```python
from build123d import *

# Parameters (mm, degrees)
ESQUISSE1_W        = 117.07
ESQUISSE1_H        = 61.3
BOSS_EXTRU_1_DEPTH = 1.6
ESQUISSE2_W        = 15
ESQUISSE2_H        = 15.6
BOSS_EXTRU_2_DEPTH = 4
ESQUISSE3_R        = 4.3
BOSS_EXTRU_3_DEPTH = 2.5


with BuildPart() as part:
    # Esquisse1 → Boss.-Extru.1 (new body)
    with BuildSketch(Plane(origin=(0, 0, 0), x_dir=(1, 0, 0), z_dir=(0, 1, 0))):
        with Locations((58.535, -30.65)):
            Rectangle(ESQUISSE1_W, ESQUISSE1_H)
    extrude(amount=BOSS_EXTRU_1_DEPTH)

    # Esquisse2 → Boss.-Extru.2 (add)
    with BuildSketch(Plane.XZ):
        with Locations((101.57, 30.8)):
            Rectangle(ESQUISSE2_W, ESQUISSE2_H)
    extrude(amount=BOSS_EXTRU_2_DEPTH)

    # Esquisse3 → Boss.-Extru.3 (add)
    with BuildSketch(Plane(origin=(0, 1.6, 0), x_dir=(1, 0, 0), z_dir=(0, 1, 0))):
        with Locations(Location((101.77, -30.65, 0), (0, 0, 270))):
            Circle(ESQUISSE3_R)
        with Locations(Location((57.27, -30.65, 0), (0, 0, 270))):
            Circle(ESQUISSE3_R)
        with Locations(Location((11.47, -30.65, 0), (0, 0, 270))):
            Circle(ESQUISSE3_R)
    extrude(amount=BOSS_EXTRU_3_DEPTH)


solid = part.part
```
The listing builds one solid part. Answer for the finished solid, in the listing's coordinates (mm). A direction names the side the tool comes from. Give positions to 0.01 mm unless a question says otherwise; leave off trailing zeros. Order: outer loops, then holes, each group sorted by start corner. A loop starts at its lowest first (then second) coordinate and runs counter-clockwise, first axis right, second up. Notation, with made-up numbers: (77.25, 54) - (100.25, 54) arc R10 cw to (100.25, 68) - close; hole circle Ø6 at (72, 82.5). An arc over 180 degrees is marked (long way). Use one line per item in the form item = value. Start each with the question number.
(1) A cutting plane is placed at B-B, the plane z = 30.65. Write down the section's boundary in (x, y).
(2) A cutting plane is placed at A-A, the plane x = 57.27. Write down the section's boundary in (y, z).
(3) A cutting plane is placed at D-D, the plane y = -2. Write down the section's boundary in (x, z).
(4) A cutting plane is placed at C-C, the plane x = 101.77. Write down the section's boundary in (y, z).
(5) Consider line 1 (X direction, y = 2, z = 32); line 2 (Y direction, x = 89, z = 12); line 3 (X direction, y = -1.5, z = 27). Determine where each line is inside the solid, lowest interval first. Write a range as from..to.
(6) Flat-ended cylindrical pins translate along their axes: pin 1 Ø10 at (x, z) = (92, 17.5) entering from +Y; pin 2 Ø1.2 at (x, y) = (104, -1) entering from +Z; pin 3 Ø3 at (x, y) = (100, -2) entering from -Z. Find the tip coordinate at first contact, or state that the pin passes through.
(7) For faces 4 (the flat face through (101, -2, 23)), 5 (the cylindrical face through (61.533, 2.832, 30.09)), 6 (the flat face through (109.07, -2, 31)), determine the directions among +Z, -Z, +X, -X, +Y, -Y from which every point of the face is accessible in a straight line to the end or side of a thin tool.
(8) The mould has two halves that part along X. Classify faces 1 (the flat face through (94.07, -2, 31)), 2 (the flat face through (57, 4.1, 31)), 3 (the cylindrical face through (105.396, 2.832, 32.962)): released by +X, released by -X, zero draft, split by the parting line, or undercut.
Ans:
q1.outline = (0, 0) - (94.07, 0) - (94.07, -4) - (109.07, -4) - (109.07, 0) - (117.07, 0) - (117.07, 1.6) - (106.07, 1.6) - (106.07, 4.1) - (97.47, 4.1) - (97.47, 1.6) - (61.57, 1.6) - (61.57, 4.1) - (52.97, 4.1) - (52.97, 1.6) - (15.77, 1.6) - (15.77, 4.1) - (7.17, 4.1) - (7.17, 1.6) - (0, 1.6) - close
q2.outline = (0, 0) - (1.6, 0) - (1.6, 26.35) - (4.1, 26.35) - (4.1, 34.95) - (1.6, 34.95) - (1.6, 61.3) - (0, 61.3) - close
q3.outline = (94.07, 23) - (109.07, 23) - (109.07, 38.6) - (94.07, 38.6) - close
q4.outline = (-4, 23) - (0, 23) - (0, 0) - (1.6, 0) - (1.6, 26.35) - (4.1, 26.35) - (4.1, 34.95) - (1.6, 34.95) - (1.6, 61.3) - (0, 61.3) - (0, 38.6) - (-4, 38.6) - close
q5.line_1 = 7.39..15.55, 53.19..61.35, 97.69..105.85
q5.line_2 = 0..1.6
q5.line_3 = 94.07..109.07
q6.pin_1 = 1.6
q6.pin_2 = 38.6
q6.pin_3 = 23
q7.face_4 = -Z, +X, -X, -Y
q7.face_5 = +Y
q7.face_6 = +Z, -Z, +X, -Y
q8.face_1 = released by -X
q8.face_2 = zero draft
q8.face_3 = undercut
